Check sheet for the modelled part. Datum: model origin and axes. Units: mm. Round coordinates to 2 decimals unless told otherwise and drop trailing zeros. Order: outer loops, then holes, each group sorted by start corner. A loop starts at its lowest first (then second) coordinate and runs counter-clockwise, first axis right, second up. Notation, with made-up numbers: (-36.75, 22) -> (-23.75, 22) arc R20 cw to (-23.75, 44) -> close; hole circle Ø10 at (-35, 20). An arc over 180 degrees is marked (long way). Use CSV: the item, a comma, the result in double quotes.
```python
from build123d import *

# Parameters (mm, degrees)
SKETCH1_R            = 7
BOSS_EXTRUDE1_DEPTH  = 130
SKETCH9_R            = 7
SKETCH9_R_2          = 3.759161882
BOSS_EXTRUDE7_DEPTH  = 5
SKETCH10_R           = 7
BOSS_EXTRUDE8_DEPTH  = 3
FILLET6_R            = 4
SKETCH12_R           = 7
SKETCH12_R_2         = 2.9
BOSS_EXTRUDE9_DEPTH  = 5
SKETCH13_R           = 7
BOSS_EXTRUDE10_DEPTH = 3
FILLET7_R            = 4
SKETCH15_R           = 7
SKETCH15_R_2         = 5.9
CUT_EXTRUDE1_DEPTH   = 20
SKETCH16_R           = 7
SKETCH16_R_2         = 5.9
CUT_EXTRUDE2_DEPTH   = 20


with BuildPart() as part:
    # Sketch1 → Boss-Extrude1 (new body, symmetric)
    with BuildSketch(Plane.XY):
        Circle(SKETCH1_R)
    extrude(amount=BOSS_EXTRUDE1_DEPTH, both=True)

    # Sketch9 → Boss-Extrude7 (add)
    with BuildSketch(Plane(origin=(0, 0, -130), x_dir=(-1, 0, 0), z_dir=(0, 0, -1))):
        Circle(SKETCH9_R)
        Circle(SKETCH9_R_2, mode=Mode.SUBTRACT)
    extrude(amount=BOSS_EXTRUDE7_DEPTH)

    # Sketch10 → Boss-Extrude8 (add)
    with BuildSketch(Plane(origin=(0, 0, -135), x_dir=(-1, 0, 0), z_dir=(0, 0, -1))):
        Circle(SKETCH10_R)
    extrude(amount=BOSS_EXTRUDE8_DEPTH)

    # Fillet6
    fillet6_edges = [part.edges().sort_by_distance(p)[0] for p in [
        (7, 0, -138),
    ]]
    fillet(fillet6_edges, radius=FILLET6_R)

    # Sketch12 → Boss-Extrude9 (add)
    with BuildSketch(Plane.XY.offset(130)):
        Circle(SKETCH12_R)
        Circle(SKETCH12_R_2, mode=Mode.SUBTRACT)
    extrude(amount=BOSS_EXTRUDE9_DEPTH)

    # Sketch13 → Boss-Extrude10 (add)
    with BuildSketch(Plane.XY.offset(135)):
        Circle(SKETCH13_R)
    extrude(amount=BOSS_EXTRUDE10_DEPTH)

    # Fillet7
    fillet7_edges = [part.edges().sort_by_distance(p)[0] for p in [
        (-7, 0, 138),
    ]]
    fillet(fillet7_edges, radius=FILLET7_R)

    # Sketch15 → Cut-Extrude1 (cut)
    with BuildSketch(Plane.XY.offset(105)):
        Circle(SKETCH15_R)
        Circle(SKETCH15_R_2, mode=Mode.SUBTRACT)
    extrude(amount=-CUT_EXTRUDE1_DEPTH, mode=Mode.SUBTRACT)

    # Sketch16 → Cut-Extrude2 (cut)
    with BuildSketch(Plane.XY.offset(-105)):
        Circle(SKETCH16_R)
        Circle(SKETCH16_R_2, mode=Mode.SUBTRACT)
    extrude(amount=CUT_EXTRUDE2_DEPTH, mode=Mode.SUBTRACT)


solid = part.part
```
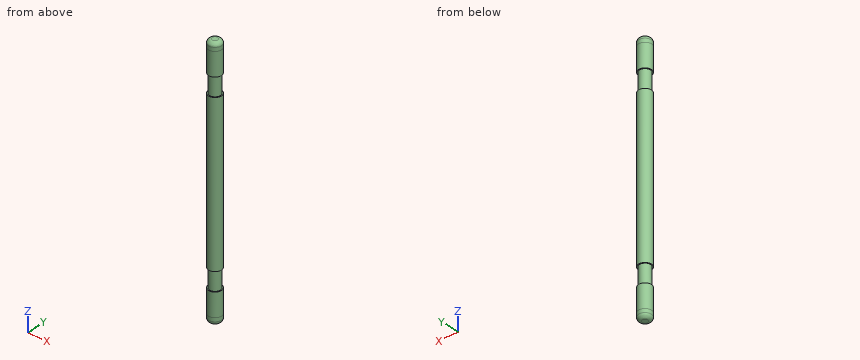
Q1. Sectioned sample at D-D, the plane z = -101. Enter the section's corners in (x, y), then the cut area to 3 significant figures.
Result sheet:
outline,"circle Ø11.8 at (0, 0)"
area,"109 mm^2"
Q2. Scan lines: L1, parallel to Z at x = -2.5, y = -0.5; L2, parallel to Y at x = 0, z = -132.3; L3, parallel to Z at x = -5, y = 3.75. Record each from-to range of solid material in increasing order.
Result sheet:
L1,"z = -138 to -135, -130 to 130, 135 to 138"
L2,"y = -7 to -3.76, 3.76 to 7"
L3,"z = -136.33 to -105, -85 to 85, 105 to 136.33"
Q3. Sectioned sample at B-B, the plane z = 111.5. Enter the section's corners in (x, y), then the cut area to 3 significant figures.
Result sheet:
outline,"circle Ø14 at (0, 0)"
area,"154 mm^2"
Q4. Sectioned sample at A-A, the plane x = 0. State how many separate pieces and enclosed holes the cut face has, then the cut area to 3 significant figures.
Result sheet:
separate pieces,"1"
enclosed holes,"2"
area,"3,700 mm^2"
Q5. Go/stop test with flat-tipped pins: pin 1 (1 mm diameter, centred on x = 4, z = 68.5, fed in from +Y); pin 2 (1.5 mm diameter, centred on y = 3.5, z = 39, fed in from -X); pin 3 (5 mm diameter, centred on y = -2, z = 93, fed in from -X). Record where each tip stops, or that it passes through.
Result sheet:
pin 1,"stops at y = 6.06"
pin 2,"stops at x = -6.44"
pin 3,"stops at x = -5.9"
